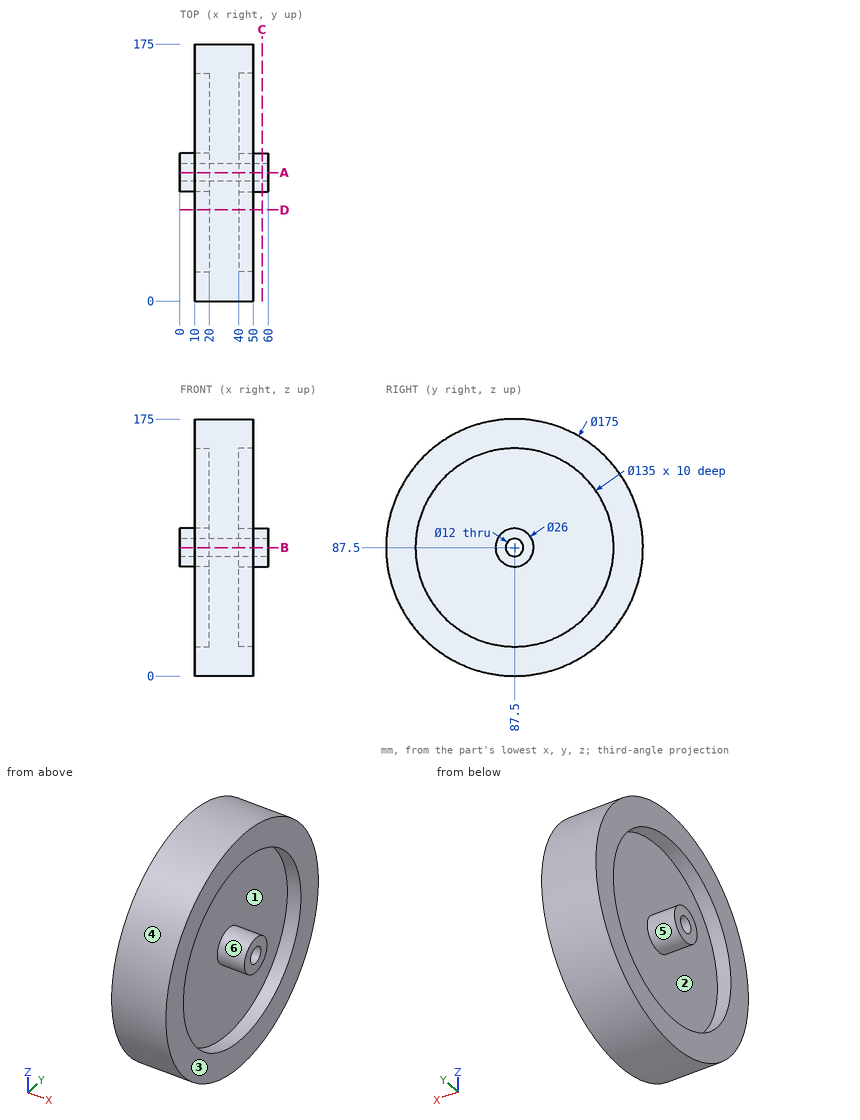
The drawing under review shows one solid part. Ordinate dimensions are in mm from its lowest x, y, z. A direction names the side the tool comes from. Coordinates: 2 decimals unless noted, no trailing zeros. Write each loop counter-clockwise with the first axis right and the second up, starting at its lowest first coordinate (ties: lowest second). Pieces come first, ordered by that corner, then holes.
1) To check wall thickness, follow L1, parallel to Y at x = 15, z = 87; L2, parallel to Y at x = 13, z = 86. State the ranges of each line that lie inside material, in increasing order.
2) Add section D-D (y = 62). Write out the cut boundary in (x, z).
3) Mouldability with a two-part tool opening along Y and no side actions: class the marked faces 3, 4, 5 and 6 as +Y half, -Y half, draft (parallel to the pull), parting line (faces both ways), or undercut.
4) Add section C-C (x = 56). Write out the cut boundary in (y, z), plus the area to 3 significant figures.
5) Insertion check: pin 1 (10 mm diameter, centred on y = 47.5, z = 119.5, fed in from +X); pin 2 (1 mm diameter, centred on x = 24.5, y = 36, fed in from -Z); pin 3 (6 mm diameter, centred on x = 28, y = 68.5, fed in from -Z); pin 4 (7 mm diameter, centred on y = 87.5, z = 87.5, fed in from +X). Each pin has a flat end and moves straight along its axis. Give the tip position at first contact, or say it passes through.
6) Add section A-A (y = 87.5). Write out the cut boundary in (x, z), plus the area to 3 significant figures.
7) Machinability: for the marked faces 1 and 2, which of the approach directions +Z, -Z, +X, -X, +Y, -Y give a long, thin tool a straight path to every point of the face, cutting with its end or side? Answer none if there is none.
Check result:
1. L1: y = 0 to 20, 74.51 to 81.52, 93.48 to 100.49, 155 to 175
1. L2: y = 0.01 to 20.02, 74.59 to 81.69, 93.31 to 100.41, 154.98 to 174.99
2. outline: (10, 3.8) - (50, 3.8) - (50, 25) - (40, 25) - (40, 150) - (50, 150) - (50, 171.2) - (10, 171.2) - (10, 150) - (20, 150) - (20, 25) - (10, 25) - close
3. face 3: draft
3. face 4: parting line
3. face 5: undercut
3. face 6: undercut
4. outline: circle Ø26 at (87.5, 87.5); hole circle Ø12 at (87.5, 87.5)
4. area: 418 mm2
5. pin 1: stops at x = 40
5. pin 2: stops at z = 16.4
5. pin 3: stops at z = 1.48
5. pin 4: passes through
6. outline: (0, 74.5) - (20, 74.5) - (20, 20) - (10, 20) - (10, 0) - (50, 0) - (50, 20) - (40, 20) - (40, 74.5) - (60, 74.5) - (60, 81.5) - (0, 81.5) - close; (0, 93.5) - (60, 93.5) - (60, 100.5) - (40, 100.5) - (40, 155) - (50, 155) - (50, 175) - (10, 175) - (10, 155) - (20, 155) - (20, 100.5) - (0, 100.5) - close
6. area: 4,620 mm2
7. face 1: +X
7. face 2: -X
